Geometry: final body of the model. Coordinates: model frame, mm. Face numbers are marked on the shaded views. A direction names the side the tool comes from. Round coordinates to 2 decimals unless told otherwise and drop trailing zeros. Order: outer loops, then holes, each group sorted by start corner. A loop starts at its lowest first (then second) coordinate and runs counter-clockwise, first axis right, second up. Notation, with made-up numbers: (4, -11) -> (52, -11) arc R20 ccw to (52, 9) -> close; hole circle Ø10 at (81.25, 11.25). An arc over 180 degrees is marked (long way). Put each result on its own line as item: value.
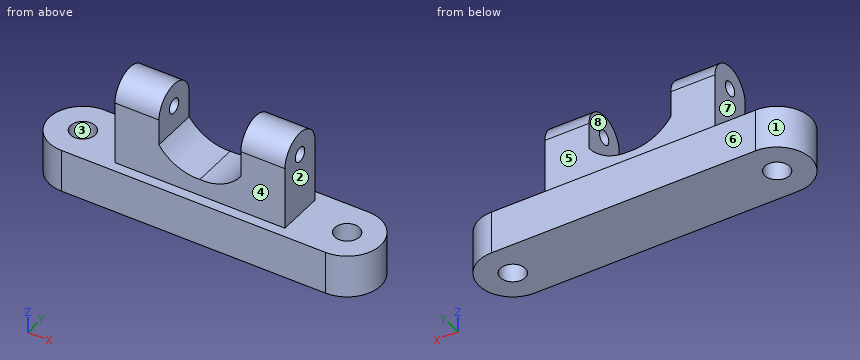
```python
from build123d import *

# Parameters (mm, degrees)
F0_R     = 10.99825
F1_DEPTH = 38.1
F3_DEPTH = 76.2
F4_R     = 6.515774
F5_DEPTH = 223.248987
F7_DEPTH = 50.806747


with BuildPart() as f1:
    # F0 (on Top) → F1 (new body)
    with BuildSketch(Plane.XY):
        with BuildLine():
            Line((117.679015, 29.866867), (0, 29.866867))
            Line((0, 29.866867), (-117.679015, 29.866867))
            ThreePointArc((-117.679015, 29.866867), (-147.545878, 4e-06), (-117.679015, -29.866859))
            Line((-117.679015, -29.866859), (0, -29.866859))
            Line((0, -29.866859), (117.679015, -29.866859))
            ThreePointArc((117.679015, -29.866859), (147.545878, 4e-06), (117.679015, 29.866867))
        make_face()
        with Locations((-117.679015, 4e-06)):
            Circle(F0_R, mode=Mode.SUBTRACT)
        with Locations((117.679015, 4e-06)):
            Circle(F0_R, mode=Mode.SUBTRACT)
    extrude(amount=F1_DEPTH)

    # F2 (on face) → F3 (join)
    with BuildSketch(Plane.XY.offset(38.1)):
        Polygon((0, 20.938881), (-75.702109, 20.938881), (-75.702109, -20.938881), (0, -20.938881), (75.702109, -20.938881), (75.702109, 20.938881), align=None)
    extrude(amount=F3_DEPTH)

    # F4 (on face) → F5 (cut, through all)
    with BuildSketch(Plane(origin=(-75.702109, 0, 0), x_dir=(0, -1, 0), z_dir=(-1, 0, 0))):
        with Locations((0, 93.864545)):
            Circle(F4_R)
        with BuildLine():
            ThreePointArc((-20.938881, 93.864545), (0, 114.228876), (20.938881, 93.864545))
            Line((20.938881, 93.864545), (20.938881, 114.3))
            Line((20.938881, 114.3), (-20.938881, 114.3))
            Line((-20.938881, 114.3), (-20.938881, 93.864545))
        make_face()
    extrude(amount=-F5_DEPTH, mode=Mode.SUBTRACT)

    # F6 (on face) → F7 (cut, through all)
    with BuildSketch(Plane.XZ.offset(20.938881)):
        with BuildLine():
            Line((36.444344, 70.606232), (36.444344, 114.3))
            Line((36.444344, 114.3), (-36.444344, 114.3))
            Line((-36.444344, 114.3), (-36.444344, 70.606232))
            ThreePointArc((-36.444344, 70.606232), (-20.505249, 57.076184), (0, 52.995533))
            ThreePointArc((0, 52.995533), (20.505249, 57.076184), (36.444344, 70.606232))
        make_face()
    extrude(amount=-F7_DEPTH, mode=Mode.SUBTRACT)


solid = f1.part
```
1. Cut plane A-A on z = 73.5. Return loops of the section in (x, y), and give its area (3 significant figures).
Ans:
outline: (-75.7, -20.94) -> (-36.44, -20.94) -> (-36.44, 20.94) -> (-75.7, 20.94) -> close; (36.44, -20.94) -> (75.7, -20.94) -> (75.7, 20.94) -> (36.44, 20.94) -> close
area: 3,290 mm²
2. Material intervals for probe 1 along X at (y, z) = (-1, 81); probe 2 along Z at (x, y) = (3, -26); probe 3 along X at (y, z) = (-5.5, 9.5), sorted ascending.
Ans:
probe 1: -75.7 to -36.44, 36.44 to 75.7
probe 2: 0 to 38.1
probe 3: -147.04 to -127.2, -108.15 to 108.15, 127.2 to 147.04
3. Cut plane C-C on z = 97. Return loops of the section in (x, y), and give its area (3 significant figures).
Ans:
outline: (-75.7, -20.61) -> (-36.44, -20.61) -> (-36.44, -5.71) -> (-75.7, -5.71) -> close; (-75.7, 5.71) -> (-36.44, 5.71) -> (-36.44, 20.61) -> (-75.7, 20.61) -> close; (36.44, -20.61) -> (75.7, -20.61) -> (75.7, -5.71) -> (36.44, -5.71) -> close; (36.44, 5.71) -> (75.7, 5.71) -> (75.7, 20.61) -> (36.44, 20.61) -> close
area: 2,340 mm²
4. Contact query for flat-ended pins moving along their axis: P1, Ø10, axis at x = 106, y = -1.5, coming from the +Z side; P2, Ø5, axis at x = -1.5, z = 49, coming from the -Y side; P3, Ø12.5, axis at y = -0.5, z = 96, coming from the -X side. Output: stop coordinate, or through.
Ans:
P1: z = 38.1
P2: y = -20.94
P3: x = -75.7
5. Draft query along Y for the marked faces 1, 2 and 3. Return one class per face: +Y half, -Y half, draft (parallel to the pull), parting line (faces both ways), or undercut.
Ans:
face 1: parting line
face 2: draft
face 3: undercut
6. Cut plane D-D on z = 32.5. Return loops of the section in (x, y).
Ans:
outline: (-117.68, -29.87) -> (117.68, -29.87) arc R29.87 ccw to (117.68, 29.87) -> (-117.68, 29.87) arc R29.87 ccw to start; hole circle Ø22 at (-117.68, 0); hole circle Ø22 at (117.68, 0)
7. Cut plane B-B on x = 62.5. Return loops of the section in (y, z), and give its area (3 significant figures).
Ans:
outline: (-29.87, 0) -> (29.87, 0) -> (29.87, 38.1) -> (20.94, 38.1) -> (20.94, 93.86) arc R20.95 ccw to (-20.94, 93.86) -> (-20.94, 38.1) -> (-29.87, 38.1) -> close; hole circle Ø13.03 at (0, 93.86)
area: 5,140 mm²
8. Set-up query: the marked faces 4, 5, 6, 7 and 8. Return all of +Z, -Z, +X, -X, +Y, -Y with unobstructed straight access to the full face (end or side cutting, diameter ignored); none if empty.
Ans:
face 4: +Z, +X, -X, -Y
face 5: +Z, +X, -X, +Y
face 6: +Z, -Z, +X, -X, +Y
face 7: +Z, -X, +Y, -Y
face 8: +Z, +Y, -Y
